Design review of the part built by this model. Coordinates are the model's own, in mm. Give positions to 0.01 mm unless a question says otherwise; leave off trailing zeros. Loops run counter-clockwise (first coordinate to the right, second up) from the corner with the lowest first, then second, coordinate; pieces in that order, holes last. Notation, with made-up numbers: M 49,55 L 67,55 A14 cw 67,65 Z; hole C 62.5,28 d11. An arc over 180 degrees is marked long. Answer as CSV lines item,"result".
Autodesk Inventor part; units mm, degrees
ref_plane "YZ Plane" through (0, 0, 0) normal (1, 0, 0) x (0, 1, 0)
ref_plane "XZ Plane" through (0, 0, 0) normal (0, 1, 0) x (-1, 0, 0)
ref_plane "XY Plane" through (0, 0, 0) normal (0, 0, 1) x (1, 0, 0)
sketch "Sketch1" plane through (0, 0, 0) normal (0, 1, 0) x (-1, 0, 0)
  line L0 (0, 0) -> (0, -172) construction
  line L1 (4, 0) -> (4, -172)
  line L2 (-4, -172) -> (-4, 0)
  arc A0 (4, 0) -> (-4, 0) centre (0, 0) ccw
  arc A1 (-4, -172) -> (4, -172) centre (0, -172) ccw
  circle A2 centre (0, 0) radius 2.1
  circle A3 centre (0, -172) radius 2.1
  circle A4 centre (7, -93) radius 2.1
  circle A5 centre (7, -93) radius 5
  circle A6 centre (-7, -150) radius 2.1
  circle A7 centre (-7, -150) radius 5
  point P0 (0, -86)
  point P1 (4, -89)
  point P2 (4, -99.3597)
  point P3 (4, -100.6403)
  point P4 (4, -97)
  point P5 (-4, -146)
  point P6 (-4, -154)
  dimension "d0" = 172
  dimension "d1" = 8
  dimension "d2" = 4.2
  dimension "d3" = 4.2
  dimension "d8" = 4.2
  dimension "d9" = 93
  dimension "d10" = 3
  dimension "d11" = 10
  dimension "d12" = 4.2
  dimension "d13" = 10
  dimension "d15" = 3
  dimension "d16" = 150
extrude "Extrusion1" add sketch "Sketch1" along normal blind 5
1. To check wall thickness, follow L1, parallel to Z at x = 0, y = 2.9; L2, parallel to X at y = 2.3, z = -172; L3, parallel to Z at x = 7, y = 4. State the ranges of each line that lie inside material, in increasing order. Write a range as [from, to].
Answer block:
L1,"[-176, -174.1], [-169.9, -2.1], [2.1, 4]"
L2,"[-4, -2.1], [2.1, 4]"
L3,"[-155, -152.1], [-147.9, -145]"
2. For P1, Ø2.5, axis at y = 2.5, z = -100.5, coming from the +X side; P2, Ø2.5, axis at y = 3, z = -61, coming from the -X side; P3, Ø4, axis at x = 0, z = 0, coming from the -Y side, all flat-tipped, find the tip position at first contact; note any pin that passes through.
Answer block:
P1,"x = 4"
P2,"x = -4"
P3,"through"
3. We need section A-A, the plane z = -150. Write out the cut boundary in (x, y).
Answer block:
outline,"M -4,0 L 4.9,0 L 4.9,5 L -4,5 Z; M 9.1,0 L 12,0 L 12,5 L 9.1,5 Z"
4. We need section B-B, the plane y = 2.9. Write out the cut boundary in (x, z).
Answer block:
outline,"M -4,-172 A4 ccw 4,-172 L 4,-154 A5 ccw long 4,-146 L 4,0 A4 ccw -4,0 L -4,-89 A5 ccw long -4,-97 Z; hole C -7,-93 d4.2; hole C 0,-172 d4.2; hole C 0,0 d4.2; hole C 7,-150 d4.2"
5. We need section C-C, the plane x = 7. Write out the cut boundary in (y, z), plus the area to 3 significant figures.
Answer block:
outline,"M 0,-155 L 5,-155 L 5,-152.1 L 0,-152.1 Z; M 0,-147.9 L 5,-147.9 L 5,-145 L 0,-145 Z"
area,"29.0 mm²"
6. We need section D-D, the plane z = -24. Write out the cut boundary in (x, y).
Answer block:
outline,"M -4,0 L 4,0 L 4,5 L -4,5 Z"
7. The part is to be moulded in two halves that separate along Z. For faces 1 (the cylindrical face through (0.273, 2.465, -174.082)), 2 (the cylindrical face through (0, 2, 4)), 3 (the flat face through (-4, 2, -44)), say which applies: pulls with the +Z half, pulls with the -Z half, needs draft (parallel to the pull), parting line crosses it, or undercut.
Answer block:
face 1,"undercut"
face 2,"pulls with the +Z half"
face 3,"needs draft"
